from build123d import *

# Parameters (mm, degrees)
F1_DEPTH = 25.4
F2_R     = 12.7
F3_DEPTH = 50.8


with BuildPart() as f1:
    # F0 (on Front) → F1 (new body)
    with BuildSketch(Plane.XZ):
        with BuildLine():
            ThreePointArc((-25.4, 50.8), (0, 25.4), (25.4, 50.8))
            Line((25.4, 50.8), (-25.4, 50.8))
        make_face()
        with BuildLine():
            Line((-25.4, 50.8), (25.4, 50.8))
            ThreePointArc((25.4, 50.8), (0, 76.2), (-25.4, 50.8))
        make_face()
        with BuildLine():
            Line((-25.4, 0), (25.4, 0))
            Line((25.4, 0), (25.4, 50.8))
            ThreePointArc((25.4, 50.8), (0, 25.4), (-25.4, 50.8))
            Line((-25.4, 50.8), (-25.4, 0))
        make_face()
    extrude(amount=F1_DEPTH)

    # F2 (on face) → F3 (cut)
    with BuildSketch(Plane.XZ.offset(25.4)):
        with Locations((0, 50.8)):
            Circle(F2_R)
    extrude(amount=-F3_DEPTH, mode=Mode.SUBTRACT)

    # F4: F1 across face


with BuildPart() as f1_1:
    add(f1.part)
    add(f1.part.mirror(Plane(origin=(0, -12.7, 0), x_dir=(1, 0, 0), z_dir=(0, 0, -1))))


solid = f1_1.part
Can you work these out from the model? Positions are in its coordinate system, mm. Give positions to 0.01 mm unless a question says otherwise; leave off trailing zeros. Loops run counter-clockwise (first coordinate to the right, second up) from the corner with the lowest first, then second, coordinate; pieces in that order, holes last. Notation, with made-up numbers: M 31,16 L 52,16 A18 ccw 52,39 Z; hole C -36,-8 d5. An arc over 180 degrees is marked long. One line per item, written item: value.
1) Imagine slicing it at A-A on x = 0. Write out the boundary of the cut face in (y, z), and give its area (3 significant figures).
Geometry check:
outline: M -25.4,-76.2 L 0,-76.2 L 0,-63.5 L -25.4,-63.5 Z; M -25.4,-38.1 L 0,-38.1 L 0,38.1 L -25.4,38.1 Z; M -25.4,63.5 L 0,63.5 L 0,76.2 L -25.4,76.2 Z
area: 2,580 mm²
2) Please list where these lines run through material, in increasing order: line 1 (Z direction, x = 0, y = -7); line 2 (Z direction, x = -11, y = -11.75); line 3 (X direction, y = -19.25, z = -49).
Geometry check:
line 1: z = -76.2 to -63.5, -38.1 to 38.1, 63.5 to 76.2
line 2: z = -73.69 to -57.15, -44.45 to 44.45, 57.15 to 73.69
line 3: x = -25.4 to -12.57, 12.57 to 25.4
3) Imagine slicing it at D-D on x = 10. Write out the boundary of the cut face in (y, z), and give its area (3 significant figures).
Geometry check:
outline: M -25.4,-74.15 L 0,-74.15 L 0,-58.63 L -25.4,-58.63 Z; M -25.4,-42.97 L 0,-42.97 L 0,42.97 L -25.4,42.97 Z; M -25.4,58.63 L 0,58.63 L 0,74.15 L -25.4,74.15 Z
area: 2,970 mm²
4) Imagine slicing it at C-C on z = 43. Write out the boundary of the cut face in (x, y).
Geometry check:
outline: M -25.4,-25.4 L -10.02,-25.4 L -10.02,0 L -25.4,0 Z; M 10.02,-25.4 L 25.4,-25.4 L 25.4,0 L 10.02,0 Z
5) Thinking about a two-plate mould opening in Z: for faces 1 (the face through (5.86, -12.878, -39.533)), 2 (the face through (0.559, -12.522, 76.194)), 3 (the face through (5.86, -12.878, 39.533)), 4 (the face through (-25.4, -13, -1)), which applies, +Z half, -Z half, draft (parallel to the pull), parting line (faces both ways), or undercut?
Geometry check:
face 1: undercut
face 2: +Z half
face 3: undercut
face 4: draft
6) I'm going to push flat-ended pins straight in: pin 1 (10 mm diameter, centred on x = -11.5, z = -54, fed in from +Y); pin 2 (1 mm diameter, centred on y = -21, z = 51.5, fed in from -X); pin 3 (5 mm diameter, centred on x = -3, y = -11.5, fed in from -Z); pin 4 (6 mm diameter, centred on x = -11, y = -16, fed in from -Z). Where does each tip first touch, or does it pass through?
Geometry check:
pin 1: stops at y = 0
pin 2: stops at x = -25.4
pin 3: stops at z = -76.2
pin 4: stops at z = -74.91
7) Imagine slicing it at B-B on y = -12. Write out the boundary of the cut face in (x, z).
Geometry check:
outline: M -25.4,-50.8 A25.4 ccw 25.4,-50.8 L 25.4,50.8 A25.4 ccw -25.4,50.8 Z; hole C 0,-50.8 d25.4; hole C 0,50.8 d25.4
